Could you check a few things on this model? Use its own coordinates, in mm. Face numbers are marked on the shaded views. Coordinates: 2 decimals unless noted, no trailing zeros. Order: outer loops, then holes, each group sorted by start corner. A loop starts at its lowest first (then second) coordinate and runs counter-clockwise, first axis right, second up. Notation, with made-up numbers: (79, 10.25) - (98, 10.25) arc R17 ccw to (98, 35.25) - close; hole circle Ø6 at (-17.75, 80). An arc over 180 degrees is marked (long way). One line per item, written item: value. Start each with the question number.
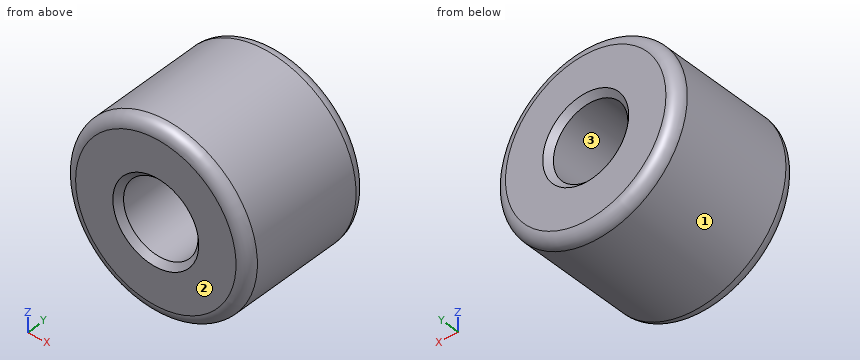
Autodesk Inventor part; units mm, degrees
ref_plane "YZ Plane" through (0, 0, 0) normal (1, 0, 0) x (0, 1, 0)
ref_plane "XZ Plane" through (0, 0, 0) normal (0, 1, 0) x (-1, 0, 0)
ref_plane "XY Plane" through (0, 0, 0) normal (0, 0, 1) x (1, 0, 0)
sketch "Sketch1" plane through (0, 0, 0) normal (0, 0, 1) x (1, 0, 0)
  line L0 (0, 6) -> (-8, 6)
  line L1 (-8, 6) -> (-8, -6)
  line L2 (-8, -6) -> (0, -6)
  line L3 (0, -6) -> (0, 6)
  line L4 (-3.25, 6) -> (-3.25, -6)
  point P0 (0, 0)
  point P1 (0, 0)
  dimension "d0" = 12
  dimension "d1" = 6.5
  dimension "d2" = 16
revolve "Revolution1" add sketch "Sketch1" angle 360 about axis through (0, -6, 0) along (0, 1, 0) contours L4 L2 L1 L0
fillet "Fillet1" radius 1 2 edges at (8, 6, 0) (8, -6, 0)
chamfer "Chamfer1" distance 0.5 angle 45 2 edges at (3.25, 6, 0) (3.25, -6, 0)
properties part number "REVO-heater" material "Rubber"
Q1. I want a section at A-A on x = 0. Please give me the cut outline in (y, z).
Q2. I want a section at C-C on y = 0.5. Please give me the cut outline in (x, z).
Q3. If I drill on L1, parallel to Z at x = 0, y = 2.25; L2, parallel to X at y = -2.5, z = -2.5; L3, parallel to Z at x = 2.75, y = -3.5, over which ranges is the centre line in solid material (lowest first)?
Q4. I'm going to push flat-ended pins straight in: pin 1 (1 mm diameter, centred on x = 3, y = 3, fed in from -Z); pin 2 (4 mm diameter, centred on y = 1.5, z = 4.5, fed in from -X); pin 3 (4 mm diameter, centred on x = 3, y = 0.5, fed in from +Z). Where does each tip first touch, or does it pass through?
Q5. We'd pull the mould along X, two halves only. Please class the marked faces 1, 2 and 3: +X half, -X half, draft (parallel to the pull), parting line (faces both ways), or undercut.
Q6. I want a section at B-B on z = 0. Please give me the cut outline in (x, y).
Values follow:
1. outline: (-6, -7) arc R1 ccw to (-5, -8) - (5, -8) arc R1 ccw to (6, -7) - (6, -3.75) - (5.5, -3.25) - (-5.5, -3.25) - (-6, -3.75) - close; (-6, 3.75) - (-5.5, 3.25) - (5.5, 3.25) - (6, 3.75) - (6, 7) arc R1 ccw to (5, 8) - (-5, 8) arc R1 ccw to (-6, 7) - close
2. outline: circle Ø16 at (0, 0); hole circle Ø6.5 at (0, 0)
3. L1: z = -8 to -3.25, 3.25 to 8
3. L2: x = -7.6 to -2.08, 2.08 to 7.6
3. L3: z = -7.51 to -1.73, 1.73 to 7.51
4. pin 1: stops at z = -7.6
4. pin 2: stops at x = -7.6
4. pin 3: stops at z = 7.94
5. face 1: parting line
5. face 2: draft
5. face 3: undercut
6. outline: (-8, -5) arc R1 ccw to (-7, -6) - (-3.75, -6) - (-3.25, -5.5) - (-3.25, 5.5) - (-3.75, 6) - (-7, 6) arc R1 ccw to (-8, 5) - close; (3.25, -5.5) - (3.75, -6) - (7, -6) arc R1 ccw to (8, -5) - (8, 5) arc R1 ccw to (7, 6) - (3.75, 6) - (3.25, 5.5) - close
